Verification items for the finished model (mm, model axes). Coordinates: 2 decimals unless noted, no trailing zeros. Order: outer loops, then holes, each group sorted by start corner. A loop starts at its lowest first (then second) coordinate and runs counter-clockwise, first axis right, second up.
Q1. Cross-section at A-A, the plane z = 3.75. Count the separate pieces of the cut face and the enclosed holes in it, and give its area (3 significant figures).
Q2. Depth check by flat-ended pin: P1, Ø5, axis at x = 10.2, y = 0, coming from the -Z side; P2, Ø5, axis at x = 10.83, y = -6.25, coming from the -Z side; P3, Ø2, axis at y = 26, z = 6.5, coming from the -X side; P4, Ø6, axis at y = -8, z = 6, coming from the -X side. Enter the tip coordinate at first touch or a pass-through.
Q3. Cross-section at C-C, the plane x = 122.5. Record the boundary of the cut face in (y, z).
Q4. Thickness scan on line 1 (Y direction, x = 150, z = 3.8); line 2 (X direction, y = -1, z = 11.5); line 3 (Y direction, x = 1.5, z = 10). Record the ranges inside material, lowest first.
Q5. Cross-section at B-B, the plane y = 25. Record the boundary of the cut face in (x, z), and give its area (3 significant figures).
from build123d import *

# Parameters (mm, degrees)
EXTRUDE_1_DEPTH           = 15
CUT_EXTRUDE_1_DEPTH       = 177.652908269
HOLE_WIZARD_1_D           = 4.3
HOLE_WIZARD_2_D           = 4.3
HOLE_WIZARD_3_D           = 4.3
HOLE_WIZARD_4_D           = 3.5
HOLE_WIZARD_4_CBORE_D     = 6.5
HOLE_WIZARD_4_CBORE_DEPTH = 1
HOLE_WIZARD_5_D           = 3.5
HOLE_WIZARD_5_CBORE_D     = 6.5
HOLE_WIZARD_5_CBORE_DEPTH = 1
HOLE_WIZARD_6_D           = 3.5
HOLE_WIZARD_6_CBORE_D     = 6.5
HOLE_WIZARD_6_CBORE_DEPTH = 1
HOLE_WIZARD_7_D           = 3.5
HOLE_WIZARD_7_CBORE_D     = 6.5
HOLE_WIZARD_7_CBORE_DEPTH = 1
HOLE_WIZARD_8_D           = 3.5
HOLE_WIZARD_8_CBORE_D     = 6.5
HOLE_WIZARD_8_CBORE_DEPTH = 1
HOLE_WIZARD_9_D           = 3.5
HOLE_WIZARD_9_CBORE_D     = 6.5
HOLE_WIZARD_9_CBORE_DEPTH = 1
HOLE_WIZARD_10_D          = 3
HOLE_WIZARD_11_D          = 3


with BuildPart() as part:
    # 草图2 → 凸台-拉伸1 (new body)
    with BuildSketch(Plane.XY.offset(15)):
        with BuildLine():
            Line((150, 22.5), (2.93516031, 34.876709047))
            ThreePointArc((2.93516031, 34.876709047), (-35, 0), (2.93516031, -34.876709047))
            Line((2.93516031, -34.876709047), (150, -22.5))
            ThreePointArc((150, -22.5), (172.5, 0), (150, 22.5))
        make_face()
    extrude(amount=-EXTRUDE_1_DEPTH)

    # 草图3 → 切除-拉伸1 (cut, through all)
    with BuildSketch(Plane(origin=(0, 0, 0), x_dir=(-1, 0, 0), z_dir=(0, 0, -1))):
        with BuildLine():
            Line((-45, 5), (-50, 5))
            ThreePointArc((-50, 5), (-55, 0), (-50, -5))
            Line((-50, -5), (-45, -5))
            ThreePointArc((-45, -5), (-40, 0), (-45, 5))
        make_face()
    extrude(amount=-CUT_EXTRUDE_1_DEPTH, mode=Mode.SUBTRACT)

    # 草图4 → 切除-旋转1 (revolve, cut)
    with BuildSketch(Plane.XZ, mode=Mode.PRIVATE) as cut_revolve_1_sk:
        Polygon((160.65, 15), (150, 15), (150, 0), (160.65, 0), (160.65, 1), (159.65, 1), (159.65, 6.2), (155.15, 6.2), (155.15, 8.8), (159.65, 8.8), (159.65, 14), (160.65, 14), align=None)
    revolve(cut_revolve_1_sk.sketch.rotate(Axis((150, 0, 15), (0, 0, -1)), 180), axis=Axis((150, 0, 15), (0, 0, -1)), mode=Mode.SUBTRACT)

    # 孔1 (through all)
    with Locations(Plane(origin=(0, 0, 0), x_dir=(-1, 0, 0), z_dir=(0, 0, -1))):
        with Locations((5.1, 8.833459119)):
            Hole(HOLE_WIZARD_1_D / 2)

    # 孔2 (through all)
    with Locations(Plane(origin=(0, 0, 0), x_dir=(-1, 0, 0), z_dir=(0, 0, -1))):
        with Locations((5.1, -8.833459119)):
            Hole(HOLE_WIZARD_2_D / 2)

    # 孔3 (through all)
    with Locations(Plane(origin=(0, 0, 0), x_dir=(-1, 0, 0), z_dir=(0, 0, -1))):
        with Locations((-10.2, 0)):
            Hole(HOLE_WIZARD_3_D / 2)

    # 孔4 (through all)
    with Locations(Plane(origin=(0, 0, 0), x_dir=(-1, 0, 0), z_dir=(0, 0, -1))):
        with Locations((10.825317547, 6.25)):
            CounterBoreHole(HOLE_WIZARD_4_D / 2, HOLE_WIZARD_4_CBORE_D / 2, HOLE_WIZARD_4_CBORE_DEPTH)

    # 孔5 (through all)
    with Locations(Plane(origin=(0, 0, 0), x_dir=(-1, 0, 0), z_dir=(0, 0, -1))):
        with Locations((0, 12.5)):
            CounterBoreHole(HOLE_WIZARD_5_D / 2, HOLE_WIZARD_5_CBORE_D / 2, HOLE_WIZARD_5_CBORE_DEPTH)

    # 孔6 (through all)
    with Locations(Plane(origin=(0, 0, 0), x_dir=(-1, 0, 0), z_dir=(0, 0, -1))):
        with Locations((-10.825317547, 6.25)):
            CounterBoreHole(HOLE_WIZARD_6_D / 2, HOLE_WIZARD_6_CBORE_D / 2, HOLE_WIZARD_6_CBORE_DEPTH)

    # 孔7 (through all)
    with Locations(Plane(origin=(0, 0, 0), x_dir=(-1, 0, 0), z_dir=(0, 0, -1))):
        with Locations((-10.825317547, -6.25)):
            CounterBoreHole(HOLE_WIZARD_7_D / 2, HOLE_WIZARD_7_CBORE_D / 2, HOLE_WIZARD_7_CBORE_DEPTH)

    # 孔8 (through all)
    with Locations(Plane(origin=(0, 0, 0), x_dir=(-1, 0, 0), z_dir=(0, 0, -1))):
        with Locations((0, -12.5)):
            CounterBoreHole(HOLE_WIZARD_8_D / 2, HOLE_WIZARD_8_CBORE_D / 2, HOLE_WIZARD_8_CBORE_DEPTH)

    # 孔9 (through all)
    with Locations(Plane(origin=(0, 0, 0), x_dir=(-1, 0, 0), z_dir=(0, 0, -1))):
        with Locations((10.825317547, -6.25)):
            CounterBoreHole(HOLE_WIZARD_9_D / 2, HOLE_WIZARD_9_CBORE_D / 2, HOLE_WIZARD_9_CBORE_DEPTH)

    # 孔10 (through all)
    with Locations(Plane(origin=(0, 0, 0), x_dir=(-1, 0, 0), z_dir=(0, 0, -1))):
        with Locations((-59, -14)):
            Hole(HOLE_WIZARD_10_D / 2)

    # 孔11 (through all)
    with Locations(Plane(origin=(0, 0, 0), x_dir=(-1, 0, 0), z_dir=(0, 0, -1))):
        with Locations((-59, 14)):
            Hole(HOLE_WIZARD_11_D / 2)


solid = part.part
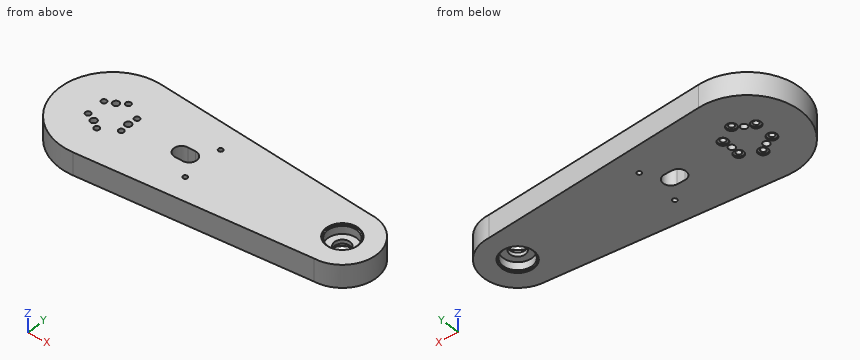
Check values:
1. separate pieces: 1
1. enclosed holes: 13
1. area: 10,800 mm2
2. P1: stops at z = 0
2. P2: stops at z = 1
2. P3: stops at x = -24.49
2. P4: stops at x = -34.64
3. outline: (-24.81, 0) - (24.81, 0) - (24.81, 15) - (-24.81, 15) - close
4. line 1: y = -22.5 to -9.65, 9.65 to 22.5
4. line 2: x = -34.99 to 8.3, 12.1 to 40.1, 54.9 to 140.4, 159.6 to 172.48
4. line 3: y = -34.97 to -13.4, -11.6 to 11.6, 13.4 to 34.97
5. outline: (-24.49, 0) - (120.29, 0) - (120.29, 15) - (-24.49, 15) - close
5. area: 2,170 mm2
